```python
from build123d import *

# Parameters (mm, degrees)
F2_R    = 1.5
F3_SIZE = 0.25


with BuildPart() as f1:
    # F0 (on Front) → F1 (revolve)
    with BuildSketch(Plane.XZ):
        Polygon((3.5, 15), (3.5, 0), (4.9, 0), (4.9, 4.048668), (7, 4.048668), (4.9, 15), align=None)
    revolve(axis=Axis((0, 0, 7.5), (0, 0, 1)))

    # F2
    f2_edges = [f1.edges().sort_by_distance(p)[0] for p in [
        (-4.9, 0, 15),
    ]]
    fillet(f2_edges, radius=F2_R)

    # F3
    f3_edges = [f1.edges().sort_by_distance(p)[0] for p in [
        (-7, 0, 4.048668),
    ]]
    chamfer(f3_edges, length=F3_SIZE)


solid = f1.part
```
Could you check a few things on this model? Use its own coordinates, in mm. A direction names the side the tool comes from. Round coordinates to 2 decimals unless told otherwise and drop trailing zeros. Write each loop counter-clockwise with the first axis right and the second up, starting at its lowest first coordinate (ties: lowest second). Pieces come first, ordered by that corner, then holes.
(1) For pin 1 (5 mm diameter, centred on x = -1.5, y = -1, fed in from -Z); pin 2 (1 mm diameter, centred on x = 5, y = 1.5, fed in from +Z); pin 3 (1 mm diameter, centred on y = 1.5, z = 8.5, fed in from -X); pin 4 (3 mm diameter, centred on x = 2, z = 2, fed in from +Y), each with a flat end and sliding along its axis, tell me the tip position at first contact or that it passes through.
Findings below:
pin 1: stops at z = 0
pin 2: stops at z = 14.56
pin 3: stops at x = -6.11
pin 4: stops at y = 4.87
(2) If I drill on probe 1 along Y at (x, z) = (-1.75, 7.5); probe 2 along Y at (x, z) = (3, 10.75); probe 3 along X at (y, z) = (-2.5, 14.25), over which ranges is the centre line in solid material (lowest first)?
Findings below:
probe 1: y = -6.09 to -3.03, 3.03 to 6.09
probe 2: y = -4.86 to -1.8, 1.8 to 4.86
probe 3: x = -4.28 to -2.45, 2.45 to 4.28
(3) Which directions (+Z, -Z, +X, -X, +Y, -Y) give clear straight access to the entire face, cutting with the end or side of a thin tool? Please do faces 1 (the face through (-4.625, -3.546, 10.159)), 2 (the face through (4, 4, 4.049)).
Findings below:
face 1: +Z
face 2: -Z
(4) Suppose I cut it at C-C on z = 2.5. Write out the boundary of the cut face in (x, y).
Findings below:
outline: circle Ø9.8 at (0, 0); hole circle Ø7 at (0, 0)
(5) Suppose I cut it at D-D on z = 13.5. Write out the boundary of the cut face in (x, y), and give its area (3 significant figures).
Findings below:
outline: circle Ø10.38 at (0, 0); hole circle Ø7 at (0, 0)
area: 46.1 mm2
(6) Thinking about a two-plate mould opening in Y: for faces 3 (the face through (3.233, -1.341, 7.395)), 4 (the face through (-1.062, -4.783, 2.053)), 5 (the face through (-2.1, -3.2, 0)), which applies, +Y half, -Y half, draft (parallel to the pull), parting line (faces both ways), or undercut?
Findings below:
face 3: undercut
face 4: parting line
face 5: draft
(7) Suppose I cut it at A-A on y = 0. Write out the boundary of the cut face in (x, z), and give its area (3 significant figures).
Findings below:
outline: (-6.95, 4.29) - (-6.75, 4.05) - (-4.9, 4.05) - (-4.9, 0) - (-3.5, 0) - (-3.5, 15) - (-3.66, 15) arc R1.5 ccw to (-5.13, 13.78) - close; (3.5, 0) - (4.9, 0) - (4.9, 4.05) - (6.75, 4.05) - (6.95, 4.29) - (5.13, 13.78) arc R1.5 ccw to (3.66, 15) - (3.5, 15) - close
area: 64.3 mm2
